```python
from build123d import *

# Parameters (mm, degrees)
F1_DEPTH = 2
F2_W     = 1.8
F2_H     = 26
F3_DEPTH = 8
F4_W     = 27.6
F4_H     = 26
F5_DEPTH = 1.8


with BuildPart() as f1:
    # F0 (on Top) → F1 (new body)
    with BuildSketch(Plane.XY):
        with BuildLine():
            Line((15.75, 18.75), (-15.75, 18.75))
            ThreePointArc((-15.75, 18.75), (-17.8713203436, 17.8713203436), (-18.75, 15.75))
            Line((-18.75, 15.75), (-18.75, -15.75))
            ThreePointArc((-18.75, -15.75), (-17.8713203436, -17.8713203436), (-15.75, -18.75))
            Line((-15.75, -18.75), (15.75, -18.75))
            ThreePointArc((15.75, -18.75), (17.8713203436, -17.8713203436), (18.75, -15.75))
            Line((18.75, -15.75), (18.75, 15.75))
            ThreePointArc((18.75, 15.75), (17.8713203436, 17.8713203436), (15.75, 18.75))
        make_face()
        with BuildLine():
            ThreePointArc((-15.25, 13.75), (-16.3106601718, 16.3106601718), (-13.75, 15.25))
            Line((-13.75, 15.25), (13.734903335, 15.25))
            ThreePointArc((13.734903335, 15.25), (15.25, 16.765096665), (16.765096665, 15.25))
            ThreePointArc((16.765096665, 15.25), (16.321335126, 14.178664874), (15.25, 13.734903335))
            Line((15.25, 13.734903335), (15.25, -13.1845953413))
            ThreePointArc((15.25, -13.1845953413), (16.7104616401, -13.7895383599), (17.3154046587, -15.25))
            ThreePointArc((17.3154046587, -15.25), (15.25, -17.3154046587), (13.1845953413, -15.25))
            Line((13.1845953413, -15.25), (-13.3112718243, -15.25))
            ThreePointArc((-13.3112718243, -15.25), (-16.6208878399, -16.6208878399), (-15.25, -13.3112718243))
            Line((-15.25, -13.3112718243), (-15.25, 13.75))
        make_face(mode=Mode.SUBTRACT)
        with BuildLine():
            Line((13.734903335, 15.25), (-13.75, 15.25))
            ThreePointArc((-13.75, 15.25), (-14.1893398282, 14.1893398282), (-15.25, 13.75))
            Line((-15.25, 13.75), (-15.25, -13.3112718243))
            ThreePointArc((-15.25, -13.3112718243), (-13.8791121601, -13.8791121601), (-13.3112718243, -15.25))
            Line((-13.3112718243, -15.25), (13.1845953413, -15.25))
            ThreePointArc((13.1845953413, -15.25), (13.7895383599, -13.7895383599), (15.25, -13.1845953413))
            Line((15.25, -13.1845953413), (15.25, 13.734903335))
            ThreePointArc((15.25, 13.734903335), (14.178664874, 14.178664874), (13.734903335, 15.25))
        make_face()
    extrude(amount=F1_DEPTH)

    # F2 (on Top) → F3 (join)
    with BuildSketch(Plane.XY):
        with Locations((-12.9, 0)):
            Rectangle(F2_W, F2_H)
        with Locations((12.9, 0)):
            Rectangle(F2_W, F2_H)
    extrude(amount=F3_DEPTH)

    # F4 (on face) → F5 (join)
    with BuildSketch(Plane.XY.offset(8)):
        Rectangle(F4_W, F4_H)
    extrude(amount=F5_DEPTH)


solid = f1.part
```
Geometry check sheet. Reference: the model listing, model coordinates, mm. A direction names the side the tool comes from. Coordinates: 2 decimals unless noted, no trailing zeros. Write each loop counter-clockwise with the first axis right and the second up, starting at its lowest first coordinate (ties: lowest second). Pieces come first, ordered by that corner, then holes. Notation, with made-up numbers: M 59.5,79.25 L 87.5,79.25 A25 ccw 87.5,103.25 Z; hole C 56.25,13.25 d5. An arc over 180 degrees is marked long. One line per item, written item: value. Start each with the question number.
(1) Tool access check on faces 1 (the face through (13.8, 0, 6)), 2 (the face through (12, 0, 5)), 3 (the face through (-0.2, -13, 8.4)), 4 (the face through (-0.2, 13, 8.4)). Record the directions out of +Z, -Z, +X, -X, +Y, -Y that give a thin tool (end or side, any length) a straight path to the whole face; none if there is none.
(2) Release check for a two-part mould opening along Z. For faces 5 (the face through (-12, 0, 5)), 6 (the face through (17.85, -17.89, 0.99)), 7 (the face through (0, 0, 9.8)) record: released by +Z, released by -Z, zero draft, split by the parting line, or undercut.
(3) Sectioned sample at B-B, the plane z = 7.5. Enter the section's corners in (x, y), and give its area (3 significant figures).
(4) Sectioned sample at D-D, the plane y = 14.5. Enter the section's corners in (x, z).
(5) Sectioned sample at A-A, the plane x = -8. Enter the section's corners in (y, z).
(6) Depth check by flat-ended pin: pin 1 (3.5 mm diameter, centred on x = -15.25, y = 15.25, fed in from +Z); pin 2 (2 mm diameter, centred on y = -7, z = 5.5, fed in from +X); pin 3 (5 mm diameter, centred on y = -5.5, z = 6, fed in from -X). Enter the tip coordinate at first touch or a pass-through.
(7) Sectioned sample at C-C, the plane y = 1.5. Enter the section's corners in (x, z).
(8) Scan lines: line 1 along Y through (x, z) = (-15.25, 0.5); line 2 along X through (y, z) = (-15.25, 0.6); line 3 along X through (y, z) = (15.25, 0.95). Record each from-to range of solid material in increasing order. Write a range as [from, to].
Filled sheet:
1. face 1: +Z, +X, +Y, -Y
1. face 2: +Y, -Y
1. face 3: +Z, +X, -X, -Y
1. face 4: +Z, +X, -X, +Y
2. face 5: undercut
2. face 6: zero draft
2. face 7: released by +Z
3. outline: M -13.8,-13 L -12,-13 L -12,13 L -13.8,13 Z; M 12,-13 L 13.8,-13 L 13.8,13 L 12,13 Z
3. area: 93.6 mm²
4. outline: M -18.75,0 L -16.55,0 L -16.55,2 L -18.75,2 Z; M -13.95,0 L 13.93,0 L 13.93,2 L -13.95,2 Z; M 16.57,0 L 18.75,0 L 18.75,2 L 16.57,2 Z
5. outline: M -18.75,0 L 18.75,0 L 18.75,2 L -18.75,2 Z; M -13,8 L 13,8 L 13,9.8 L -13,9.8 Z
6. pin 1: z = 2
6. pin 2: x = 13.8
6. pin 3: x = -13.8
7. outline: M -18.75,0 L 18.75,0 L 18.75,2 L 13.8,2 L 13.8,9.8 L -13.8,9.8 L -13.8,2 L -18.75,2 Z; hole M -12,2 L 12,2 L 12,8 L -12,8 Z
8. line 1: [-18.75, -17.19], [-13.31, 13.75], [16.75, 18.75]
8. line 2: [-18.75, -17.19], [-13.31, 13.18], [17.32, 18.75]
8. line 3: [-18.75, -16.75], [-13.75, 13.73], [16.77, 18.75]
